Autodesk Fusion 360 part; units mm, degrees
sketch "Skizze1" plane through (0, 0, 0) normal (0, 0, 1) x (1, 0, 0)
  line L0 (0, 0) -> (95, 0)
  line L1 (95, 0) -> (95, 66)
  line L2 (95, 66) -> (0, 66)
  line L3 (0, 66) -> (0, 0)
  line L4 (47.5, 0) -> (47.5, 66) construction
  line L5 (0, 33) -> (95, 33) construction
  line L6 (90, 61) -> (5, 61)
  line L7 (5, 61) -> (5, 5)
  line L8 (5, 5) -> (90, 5)
  line L9 (90, 5) -> (90, 61)
  line L10 (90, 61) -> (5, 5) construction
  line L11 (5, 61) -> (90, 5) construction
  line L12 (5, 61) -> (8.5, 61)
  line L13 (8.5, 61) -> (8.5, 57.5)
  line L14 (8.5, 57.5) -> (5, 57.5)
  line L15 (5, 57.5) -> (5, 61)
  circle A0 centre (8.5, 57.5) radius 2.5
  line L16 (5, 5) -> (8.5, 5)
  line L17 (8.5, 5) -> (8.5, 8.5)
  line L18 (8.5, 8.5) -> (5, 8.5)
  line L19 (5, 8.5) -> (5, 5)
  circle A1 centre (8.5, 8.5) radius 2.5
  line L20 (8.5, 8.5) -> (66.5, 8.5)
  circle A2 centre (66.5, 8.5) radius 2.5
  line L21 (8.5, 57.5) -> (66.5, 57.5)
  circle A3 centre (66.5, 57.5) radius 2.5
  point P0 (47.5, 33)
  dimension "d1" = 95
  dimension "d2" = 66
  dimension "d3" = 85
  dimension "d4" = 56
  dimension "d5" = 3.5
  dimension "d6" = 3.5
  dimension "d7" = 5
  dimension "d8" = 3.5
  dimension "d9" = 3.5
  dimension "d10" = 5
  dimension "d11" = 58
  dimension "d12" = 5
  dimension "d13" = 58
  dimension "d14" = 5
extrude "Extrusion1" add sketch "Skizze1" along normal blind 2 contours L0 L1 L2 L3 | L6 L7 L8 L9 L13 L14 A0 L17 L18 A1 | L6 L7 L12 L13 L14 L15 A0 | L7 L8 L16 L17 L18 L19 A1
extrude "Extrusion2" add sketch "Skizze1" along normal blind 12 contours A3 | A2 | L13 A0 L21 | L13 L14 A0 | L14 A0 L21 | L17 L18 A1 | L17 A1 L20 | L18 A1 L20
sketch "Skizze2" plane through (0, 0, 12) normal (0, 0, 1) x (-1, 0, 0)
  circle A0 centre (-8.5, -57.5) radius 2.5
  circle A1 centre (-8.5, -57.5) radius 1
  dimension "d19" = 2
extrude "Extrusion3" cut sketch "Skizze2" against normal blind 10 contours A1
sketch "Skizze3" plane through (0, 0, 12) normal (0, 0, 1) x (-1, 0, 0)
  circle A0 centre (-8.5, -8.5) radius 2.5
  circle A1 centre (-8.5, -8.5) radius 1
  dimension "d22" = 2
extrude "Extrusion4" cut sketch "Skizze3" against normal blind 10 contours A1
sketch "Skizze4" plane through (0, 0, 12) normal (0, 0, 1) x (-1, 0, 0)
  circle A0 centre (-66.5, -8.5) radius 2.5
  circle A1 centre (-66.5, -8.5) radius 1
  dimension "d25" = 2
extrude "Extrusion5" cut sketch "Skizze4" against normal blind 10 contours A1
sketch "Skizze5" plane through (0, 0, 12) normal (0, 0, 1) x (-1, 0, 0)
  circle A0 centre (-66.5, -57.5) radius 2.5
  circle A1 centre (-66.5, -57.5) radius 1
  dimension "d28" = 2
extrude "Extrusion6" cut sketch "Skizze5" against normal blind 10 contours A1
extrude "Extrusion7" cut 4 faces at (8.8074, 8.4503, 2) (8.2374, 57.0304, 2) (66.1815, 58.0517, 2) (66.5787, 9.0963, 2) along direction (0, 0, -1) blind 1
sketch "Skizze6" plane through (0, 0, 2) normal (0, 0, 1) x (-1, 0, 0)
  circle A0 centre (-66.5, -57.5) radius 2.5
  circle A1 centre (-8.5, -8.5) radius 2.5
  circle A2 centre (-8.5, -57.5) radius 2.5
  circle A3 centre (-66.5, -8.5) radius 2.5
  line L0 (0, -66) -> (0, 0)
  line L1 (0, 0) -> (-95, 0)
  line L2 (-95, 0) -> (-95, -66)
  line L3 (-95, -66) -> (0, -66)
  circle A4 centre (-8.5, -57.5) radius 3.5
  circle A5 centre (-66.5, -57.5) radius 3.5
  circle A6 centre (-8.5, -8.5) radius 3.5
  dimension "d33" = 7
  dimension "d34" = 7
  dimension "d35" = 7
extrude "Extrusion8" cut sketch "Skizze1" along normal blind 2 contours L0 L1 L2 L3
extrude "Extrusion9" cut 1 faces at (90, 23.6667, 0.6667) along direction (-1, 0, 0) blind 20
fillet "Abrundung1" radius 3.5 4 edges at (5, 5, 1) (70, 5, 1) (70, 61, 1) (5, 61, 1)
Check sheet for the modelled part. Datum: model origin and axes. Units: mm. A direction names the side the tool comes from. Round coordinates to 2 decimals unless told otherwise and drop trailing zeros. Order: outer loops, then holes, each group sorted by start corner. A loop starts at its lowest first (then second) coordinate and runs counter-clockwise, first axis right, second up.
(1) Go/stop test with flat-tipped pins: P1, Ø3, axis at x = 26.5, y = 36.5, coming from the +Z side; P2, Ø0.6, axis at x = 66.5, y = 9, coming from the +Z side. Record where each tip stops, or that it passes through.
(2) Access from +Z, -Z, +X, -X, +Y, -Y to the whole of each face (thin tool, end or side, straight path). Record for faces 4 (the cylindrical face through (9.84, 55.39, 6.93)), 5 (the flat face through (37, 33, 0)).
(3) Cross-section at C-C, the plane y = 42.5. Enter the section's corners in (x, z).
(4) Cross-section at A-A, the plane z = 10.75. Enter the section's corners in (x, y).
(5) Draft check along Y on faces 1 (the cylindrical face through (7.96, 56.66, 6.58)), 2 (the flat face through (8, 7, 12)), 3 (the flat face through (38, 61, 1)). Enter one of: pulls with the +Y half, pulls with the -Y half, needs draft (parallel to the pull), parting line crosses it, or undercut.
(6) Cross-section at B-B, the plane x = 31.5. Enter the section's corners in (y, z), and give its area (3 significant figures).
(7) Scan lines: probe 1 along X at (y, z) = (57.5, 8.5); probe 2 along Y at (x, z) = (66.5, 4.75); probe 3 along Z at (x, y) = (46.5, 18). Record each from-to range of solid material in increasing order.
Check sheet entries:
1. P1: stops at z = 2
1. P2: stops at z = 1
2. face 4: +Z
2. face 5: -Z, +X, -X, +Y, -Y
3. outline: (5, 0) - (70, 0) - (70, 2) - (5, 2) - close
4. outline: circle Ø5 at (8.5, 8.5); circle Ø5 at (8.5, 57.5); circle Ø5 at (66.5, 8.5); circle Ø5 at (66.5, 57.5); hole circle Ø2 at (8.5, 8.5); hole circle Ø2 at (8.5, 57.5); hole circle Ø2 at (66.5, 8.5); hole circle Ø2 at (66.5, 57.5)
5. face 1: undercut
5. face 2: needs draft
5. face 3: pulls with the +Y half
6. outline: (5, 0) - (61, 0) - (61, 2) - (5, 2) - close
6. area: 112 mm2
7. probe 1: x = 6 to 7.5, 9.5 to 11, 64 to 65.5, 67.5 to 69
7. probe 2: y = 6 to 7.5, 9.5 to 11, 55 to 56.5, 58.5 to 60
7. probe 3: z = 0 to 2
